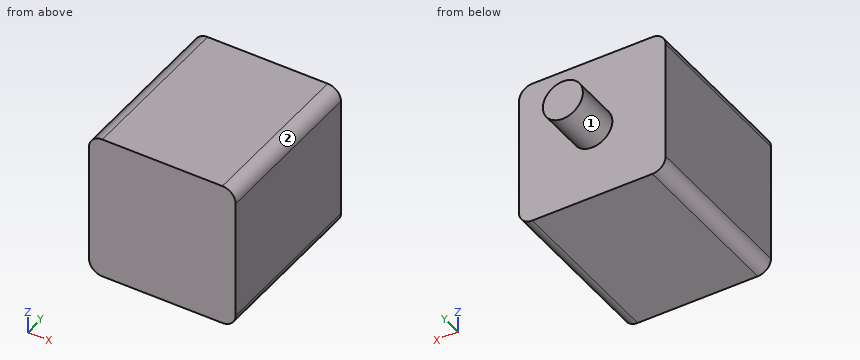
from build123d import *

# Parameters (mm, degrees)
SKETCH1_R           = 6
BOSS_EXTRUDE1_DEPTH = 25
SKETCH2_R           = 3
BOSS_EXTRUDE2_DEPTH = 7


with BuildPart() as part:
    # Sketch1 → Boss-Extrude1 (new body)
    with BuildSketch(Plane(origin=(0, 0, 0), x_dir=(1, 0, 0), z_dir=(0, 1, 0))):
        with BuildLine():
            ThreePointArc((-11, 9), (-10.414213562, 10.414213562), (-9, 11))
            Line((-9, 11), (9, 11))
            ThreePointArc((9, 11), (10.414213562, 10.414213562), (11, 9))
            Line((11, 9), (11, -9))
            ThreePointArc((11, -9), (10.414213562, -10.414213562), (9, -11))
            Line((9, -11), (-9, -11))
            ThreePointArc((-9, -11), (-10.414213562, -10.414213562), (-11, -9))
            Line((-11, -9), (-11, 9))
        make_face()
        Circle(SKETCH1_R, mode=Mode.SUBTRACT)
        Circle(SKETCH1_R)
    extrude(amount=BOSS_EXTRUDE1_DEPTH)

    # Sketch2 → Boss-Extrude2 (add)
    with BuildSketch(Plane(origin=(0, 25, 0), x_dir=(1, 0, 0), z_dir=(0, 1, 0))):
        with Locations(Location((0, 0, 0), (0, 0, 270))):
            Circle(SKETCH2_R)
    extrude(amount=BOSS_EXTRUDE2_DEPTH)


solid = part.part
Check sheet for the modelled part. Datum: model origin and axes. Units: mm. Face numbers are marked on the shaded views. A direction names the side the tool comes from. Give positions to 0.01 mm unless a question says otherwise; leave off trailing zeros. Write each loop counter-clockwise with the first axis right and the second up, starting at its lowest first coordinate (ties: lowest second). Pieces come first, ordered by that corner, then holes. Notation, with made-up numbers: (38, -36.5) -> (62, -36.5) arc R14 cw to (62, -16.5) -> close; hole circle Ø4 at (36.5, 46). An arc over 180 degrees is marked (long way). Use one line per item in the form item = value. Start each with the question number.
1. Section check A-A (x = 0). Record the cut outline in (y, z).
2. Section check C-C (x = -8.5). Record the cut outline in (y, z), and give its area (3 significant figures).
3. Section check D-D (z = -3.75). Record the cut outline in (x, y), and give its area (3 significant figures).
4. Go/stop test with a flat-tipped pin: P1, Ø1.5, axis at x = -8.5, z = -2.5, coming from the +Y side. Record where the tip stops, or that it passes through.
5. Thickness scan on line 1 along Y through (x, z) = (6.5, -1.25); line 2 along X through (y, z) = (23, 9.5); line 3 along Z through (x, y) = (-9.75, 21). Record the ranges inside material, lowest first. Write a range as from..to.
6. Section check B-B (z = 0). Record the cut outline in (x, y).
7. Access from +Z, -Z, +X, -X, +Y, -Y to the whole of each face (thin tool, end or side, straight path). Record for the marked faces 1 and 2.
Conclusion:
q1.outline = (0, -11) -> (25, -11) -> (25, -3) -> (32, -3) -> (32, 3) -> (25, 3) -> (25, 11) -> (0, 11) -> close
q2.outline = (0, -11) -> (25, -11) -> (25, 11) -> (0, 11) -> close
q2.area = 550 mm²
q3.outline = (-11, 0) -> (11, 0) -> (11, 25) -> (-11, 25) -> close
q3.area = 550 mm²
q4.P1 = 25
q5.line_1 = 0..25
q5.line_2 = -10.94..10.94
q5.line_3 = -10.85..10.85
q6.outline = (-11, 0) -> (11, 0) -> (11, 25) -> (3, 25) -> (3, 32) -> (-3, 32) -> (-3, 25) -> (-11, 25) -> close
q7.face_1 = +Y
q7.face_2 = +Z, +X, +Y, -Y
